Verification items for this drawing (mm, ordinates from the low corner). Round coordinates to 2 decimals unless told otherwise and drop trailing zeros. Write each loop counter-clockwise with the first axis right and the second up, starting at its lowest first coordinate (ties: lowest second). Pieces come first, ordered by that corner, then holes. Notation, with made-up numbers: (82.25, -13) -> (98.25, -13) arc R9 ccw to (98.25, -7) -> close; hole circle Ø11 at (61.5, 43). An arc over 180 degrees is marked (long way). Return JSON: item names as keys, results as strings. Group by question number.
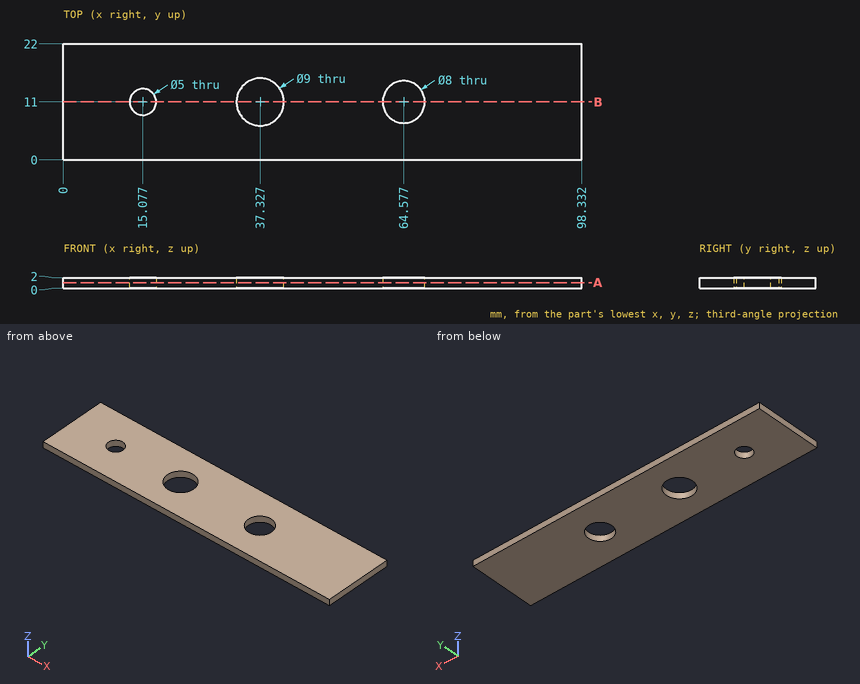
1) Sectioned sample at B-B on y = 11. Enter the section's corners in (x, z).
2) Sectioned sample at A-A on z = 1.1. Enter the section's corners in (x, y).
3) Material ranges on probe 1 along X at (y, z) = (13.25, 0.45) (1 decimal); probe 2 along X at (y, z) = (9.5, 1.1) (1 decimal); probe 3 along X at (y, z) = (13.75, 0.35) (1 decimal), recorded low to high. Write a range as [from, to].
Evaluation:
{
 "1": {"outline": "(0, 0) -> (12.58, 0) -> (12.58, 2) -> (0, 2) -> close; (17.58, 0) -> (32.83, 0) -> (32.83, 2) -> (17.58, 2) -> close; (41.83, 0) -> (60.58, 0) -> (60.58, 2) -> (41.83, 2) -> close; (68.58, 0) -> (98.33, 0) -> (98.33, 2) -> (68.58, 2) -> close"},
 "2": {"outline": "(0, 0) -> (98.33, 0) -> (98.33, 22) -> (0, 22) -> close; hole circle Ø5 at (15.08, 11); hole circle Ø9 at (37.33, 11); hole circle Ø8 at (64.58, 11)"},
 "3": {"probe 1": "x = [0, 14], [16.2, 33.4], [41.2, 61.3], [67.9, 98.3]", "probe 2": "x = [0, 13.1], [17.1, 33.1], [41.6, 60.9], [68.3, 98.3]", "probe 3": "x = [0, 33.8], [40.9, 61.7], [67.5, 98.3]"}
}
